from build123d import *

# Parameters (mm, degrees)
SKETCH_1_R      = 5
EXTRUDE_1_DEPTH = 24
CHAMFER_1_SIZE  = 1
SKETCH_6_W      = 2.5
SKETCH_6_H      = 5


with BuildPart() as part:
    # ｽｹｯﾁ1 → ﾎﾞｽ - 押し出し1 (new, symmetric)
    with BuildSketch(Plane.XY):
        Circle(SKETCH_1_R)
    extrude(amount=EXTRUDE_1_DEPTH, both=True)

    # 面取り1
    chamfer_1_edges = [part.edges().sort_by_distance(p)[0] for p in [
        (-5, 0, -24),
        (-5, 0, 24),
    ]]
    chamfer(chamfer_1_edges, length=CHAMFER_1_SIZE)

    # ｽｹｯﾁ6 → M6x1.0 ねじ穴用ねじ下穴ﾄﾞﾘﾙ1 (revolve, cut)
    with BuildSketch(Plane(origin=(0, 0, 17.8), x_dir=(0, 0, 1), z_dir=(0, 1, 0))):
        with Locations((1.25, 2.5)):
            Rectangle(SKETCH_6_W, SKETCH_6_H)
    m6x1_0_1 = revolve(axis=Axis((-6.35, 0, 17.8), (1, 0, 0)), mode=Mode.SUBTRACT)

    # ﾐﾗｰ1: M6x1.0 ねじ穴用ねじ下穴ﾄﾞﾘﾙ1 across plane
    add(m6x1_0_1.mirror(Plane(origin=(0, 0, 0), x_dir=(0, 0, 1), z_dir=(1, 0, 0))), mode=Mode.SUBTRACT)


solid = part.part
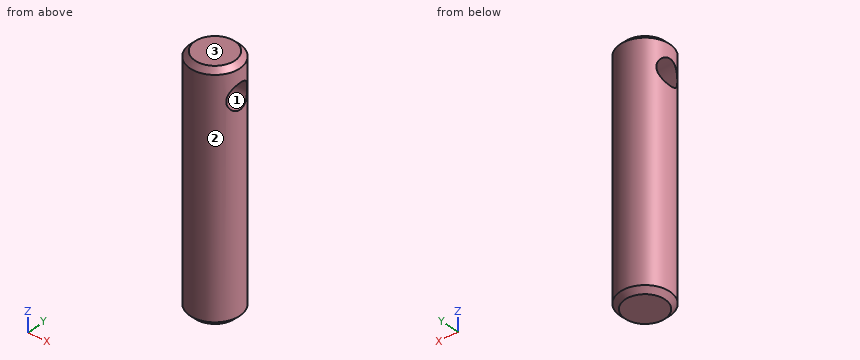
The listing builds one solid part. Answer for the finished solid, in the listing's coordinates (mm). Face numbers are marked on the shaded views. Round coordinates to 2 decimals unless told otherwise and drop trailing zeros. Order: outer loops, then holes, each group sorted by start corner. A loop starts at its lowest first (then second) coordinate and runs counter-clockwise, first axis right, second up. Notation, with made-up numbers: (75.5, -31) -> (122.5, -31) arc R21 cw to (122.5, -23) -> close; hole circle Ø5 at (-5, -17.5). An arc over 180 degrees is marked (long way). One line per item, written item: value.
Item 1: Find section B-B, the plane x = 0. Give the vertices of the cut face in (y, z).
Taken from the geometry:
outline: (-5, -23) -> (-4, -24) -> (4, -24) -> (5, -23) -> (5, 23) -> (4, 24) -> (-4, 24) -> (-5, 23) -> close; hole circle Ø5 at (0, 17.8)
Item 2: For a pull along Y with two mould halves and no side action, classify the marked faces 1, 2 and 3 as released by +Y, released by -Y, zero draft, split by the parting line, or undercut.
Taken from the geometry:
face 1: undercut
face 2: split by the parting line
face 3: zero draft
Item 3: Find section C-C, the plane z = 17.8. Give the vertices of the cut face in (x, y).
Taken from the geometry:
outline: (-4.33, -2.5) arc R5 ccw to (4.33, -2.5) -> close; (-4.33, 2.5) -> (4.33, 2.5) arc R5 ccw to start
Item 4: Find section D-D, the plane z = 10.5. Give the vertices of the cut face in (x, y).
Taken from the geometry:
outline: circle Ø10 at (0, 0)
Item 5: Straight lines are drawn through the part: L1, parallel to Z at x = -1.5, y = 0; L2, parallel to Z at x = -4, y = -1.25; L3, parallel to Y at x = -1, z = 17.8. For each, find the intervals that lie inside material, in ascending order.
Taken from the geometry:
L1: z = -24 to 15.3, 20.3 to 24
L2: z = -23.81 to 15.63, 19.97 to 23.81
L3: y = -4.9 to -2.5, 2.5 to 4.9
Item 6: Find section A-A, the plane y = 0. Give the vertices of the cut face in (x, z), then the cut area to 3 significant figures.
Taken from the geometry:
outline: (-5, -23) -> (-4, -24) -> (4, -24) -> (5, -23) -> (5, 15.3) -> (-5, 15.3) -> close; (-5, 20.3) -> (5, 20.3) -> (5, 23) -> (4, 24) -> (-4, 24) -> (-5, 23) -> close
area: 428 mm2
Item 7: Given P1, Ø3, axis at y = -3, z = -12, coming from the -X side; P2, Ø3, axis at y = 3, z = 4, coming from the +X side, each flat-ended and moving along its own axis, determine where each tip first touches the part or whether it passes through.
Taken from the geometry:
P1: stops at x = -4.77
P2: stops at x = 4.77
